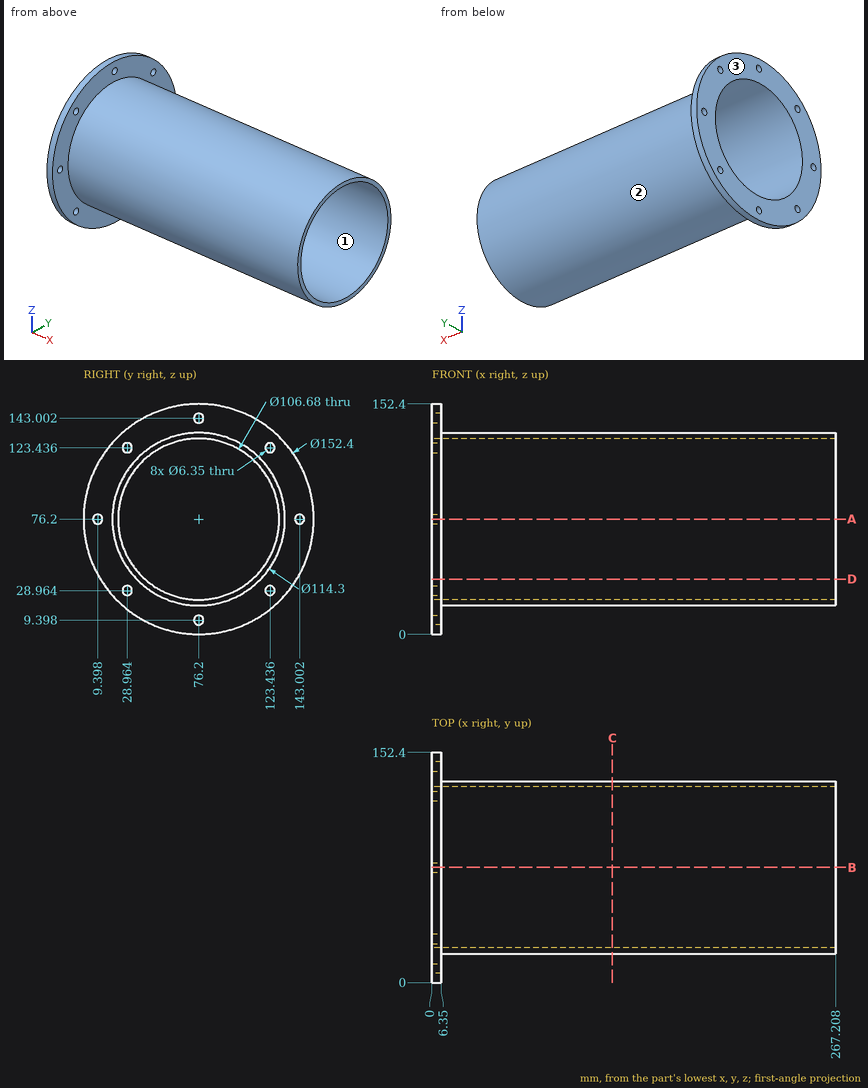
Verification items for this drawing (mm, ordinates from the low corner). Coordinates: 2 decimals unless noted, no trailing zeros. Order: outer loops, then holes, each group sorted by start corner. A loop starts at its lowest first (then second) coordinate and runs counter-clockwise, first axis right, second up. Notation, with made-up numbers: (51, 30) - (64, 30) arc R30 cw to (64, 64) - close; hole circle Ø1 at (12.25, 38). An arc over 180 degrees is marked (long way). Answer in a Markdown table with one row per item. Add a question column.
1. Section check C-C (x = 119.5). Enter the section's corners in (y, z).
2. Section check D-D (z = 36.5). Enter the section's corners in (x, y), plus the area to 3 significant figures.
3. Material ranges on L1, parallel to Y at x = 93, z = 75; L2, parallel to Z at x = 145, y = 76; L3, parallel to X at y = 137, z = 110, recorded low to high. Write a range as [from, to].
4. Section check A-A (z = 76.2). Enter the section's corners in (x, y), plus the area to 3 significant figures.
5. Draft check along Y on the marked faces 1, 2 and 3. Enter one of: +Y half, -Y half, draft (parallel to the pull), parting line (faces both ways), or undercut.
6. Gauge pin test, flat ends, axial feed: pin 1 Ø5 at (y, z) = (76.2, 143.002) entering from -X; pin 2 Ø8 at (x, y) = (151, 58) entering from +Z; pin 3 Ø8 at (x, z) = (31, 104) entering from -Y; pin 4 Ø3 at (x, z) = (218, 28.5) entering from +Y. Record the tip position at first contact, or that the pin passes through.
Data:
| question | item | result |
|---|---|---|
| 1 | outline | circle Ø114.3 at (76.2, 76.2); hole circle Ø106.68 at (76.2, 76.2) |
| 2 | outline | (0, 11.16) - (6.35, 11.16) - (6.35, 35.09) - (267.21, 35.09) - (267.21, 40.58) - (0, 40.58) - close; (0, 111.82) - (267.21, 111.82) - (267.21, 117.31) - (6.35, 117.31) - (6.35, 141.24) - (0, 141.24) - close |
| 2 | area | 3,240 mm² |
| 3 | L1 | y = [19.06, 22.87], [129.53, 133.34] |
| 3 | L2 | z = [19.05, 22.86], [129.54, 133.35] |
| 3 | L3 | x = [0, 6.35] |
| 4 | outline | (0, 0) - (6.35, 0) - (6.35, 6.22) - (0, 6.22) - close; (0, 12.57) - (6.35, 12.57) - (6.35, 19.05) - (267.21, 19.05) - (267.21, 22.86) - (0, 22.86) - close; (0, 129.54) - (267.21, 129.54) - (267.21, 133.35) - (6.35, 133.35) - (6.35, 139.83) - (0, 139.83) - close; (0, 146.18) - (6.35, 146.18) - (6.35, 152.4) - (0, 152.4) - close |
| 4 | area | 2,200 mm² |
| 5 | face 1 | undercut |
| 5 | face 2 | parting line |
| 5 | face 3 | draft |
| 6 | pin 1 | passes through |
| 6 | pin 2 | stops at z = 131.56 |
| 6 | pin 3 | stops at y = 24.24 |
| 6 | pin 4 | stops at y = 109.84 |
